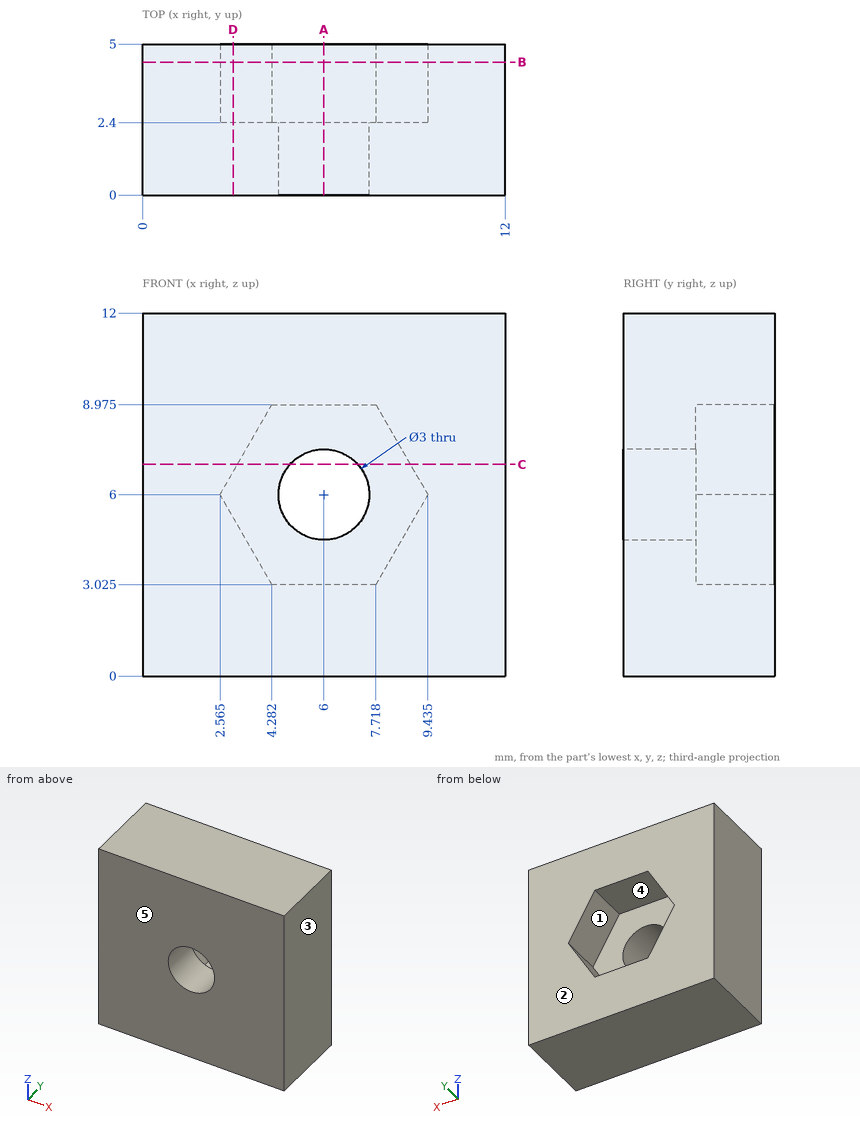
For this review, use the dimensioned drawing (mm, ordinates from the lowest corner) and the shaded views. A direction names the side the tool comes from. Round coordinates to 2 decimals unless told otherwise and drop trailing zeros. Write each loop counter-clockwise with the first axis right and the second up, starting at its lowest first coordinate (ties: lowest second). Pieces come first, ordered by that corner, then holes. Notation, with made-up numbers: (-13.75, -17) -> (43.25, -17) arc R19 ccw to (43.25, 16) -> close; hole circle Ø11 at (1, 15.5). An arc over 180 degrees is marked (long way). Use CSV: the item, a comma, the result in double quotes.
Q1. Consider section D-D (x = 3). Give the boundary of the cut face in (y, z).
Checks:
outline,"(0, 0) -> (5, 0) -> (5, 5.25) -> (2.4, 5.25) -> (2.4, 6.75) -> (5, 6.75) -> (5, 12) -> (0, 12) -> close"
Q2. For the marked faces 1 and 2, list the 3-axis set-ups (+Z, -Z, +X, -X, +Y, -Y) from which the entire face can be reached by the end or side of a thin tool; tool diameter is ignored.
Checks:
face 1,"+Y"
face 2,"+Z, -Z, +X, -X, +Y"
Q3. For pin 1 Ø1 at (y, z) = (2.5, 2.5) entering from -X, flat-tipped, find the tip position at first contact; note if it passes through.
Checks:
pin 1,"x = 0"
Q4. To check wall thickness, follow probe 1 along X at (y, z) = (1.8, 6); probe 2 along Z at (x, y) = (4.5, 4.45) (1 decimal); probe 3 along Z at (x, y) = (6.25, 1.65). State the ranges of each line that lie inside material, in increasing order. Write a range as [from, to].
Checks:
probe 1,"[0, 4.5], [7.5, 12]"
probe 2,"[0, 3], [9, 12]"
probe 3,"[0, 4.52], [7.48, 12]"
Q5. Consider section C-C (z = 7). Give the boundary of the cut face in (x, y).
Checks:
outline,"(0, 0) -> (4.88, 0) -> (4.88, 2.4) -> (3.14, 2.4) -> (3.14, 5) -> (0, 5) -> close; (7.12, 0) -> (12, 0) -> (12, 5) -> (8.86, 5) -> (8.86, 2.4) -> (7.12, 2.4) -> close"
Q6. Mouldability with a two-part tool opening along X and no side actions: class the marked faces 3, 4 and 5 as released by +X, released by -X, zero draft, split by the parting line, or undercut.
Checks:
face 3,"released by +X"
face 4,"undercut"
face 5,"zero draft"
Q7. Consider section B-B (y = 4.4). Give the boundary of the cut face in (x, z) (1 decimal).
Checks:
outline,"(0, 0) -> (12, 0) -> (12, 12) -> (0, 12) -> close; hole (2.6, 6) -> (4.3, 3) -> (7.7, 3) -> (9.4, 6) -> (7.7, 9) -> (4.3, 9) -> close"
Q8. Consider section A-A (x = 6). Give the boundary of the cut face in (y, z) (1 decimal).
Checks:
outline,"(0, 0) -> (5, 0) -> (5, 3) -> (2.4, 3) -> (2.4, 4.5) -> (0, 4.5) -> close; (0, 7.5) -> (2.4, 7.5) -> (2.4, 9) -> (5, 9) -> (5, 12) -> (0, 12) -> close"
